Source: CAD feature listing. Evaluate the final solid. Frame: model axes, mm. A direction names the side the tool comes from. Give positions to 0.01 mm unless a question says otherwise; leave off trailing zeros. Loops run counter-clockwise (first coordinate to the right, second up) from the corner with the lowest first, then second, coordinate; pieces in that order, holes last. Notation, with made-up numbers: (-33, 66.25) - (-23, 66.25) arc R13 cw to (-23, 78.25) - close; hole circle Ø5 at (-10.5, 3.5). An arc over 180 degrees is marked (long way). Put each result on its own line as item: value.
Autodesk Inventor part; units mm, degrees
ref_plane "YZ Plane" through (0, 0, 0) normal (1, 0, 0) x (0, 1, 0)
ref_plane "XZ Plane" through (0, 0, 0) normal (0, 1, 0) x (-1, 0, 0)
ref_plane "XY Plane" through (0, 0, 0) normal (0, 0, 1) x (1, 0, 0)
sketch "Boceto1" plane through (0, 0, 0) normal (0, 1, 0) x (-1, 0, 0)
  circle A0 centre (0, 0) radius 30
  circle A1 centre (0, 0) radius 35
  dimension "d0" = 60
  dimension "d1" = 70
extrude "Extrusión1" add sketch "Boceto1" along normal blind 100
sketch "Boceto2" plane through (0, 0, 0) normal (0, -1, 0) x (1, 0, 0)
  line L0 (0, 0) -> (0, 45)
  line L1 (45, 35) -> (45, -35)
  line L2 (40, 35) -> (40, -35)
  line L3 (45, 0) -> (45, -35)
  line L4 (45, -35) -> (40, -35)
  line L5 (45, 0) -> (45, 35)
  line L6 (45, 35) -> (40, 35)
extrude "Extrusión2" add sketch "Boceto2" against normal blind 35
sketch "Boceto3" plane through (45, 0, 35) normal (1, 0, 0) x (0, 0, -1)
  line L0 (35, 0) -> (35, 35)
  circle A0 centre (35, 35) radius 35
  line L1 (0, 0) -> (0, 35)
  line L2 (0, 35) -> (0, 0)
  line L3 (70, 0) -> (0, 0)
  line L4 (0, 0) -> (70, 0)
  line L5 (70, 0) -> (70, 35)
  line L6 (70, 0) -> (70, 35)
  point P0 (70, 35)
extrude "Extrusión3" cut sketch "Boceto3" against normal blind 100 contours L5 L3 A0 | A0 L3 L1
sketch "Boceto4" plane through (45, 35, 0) normal (1, 0, 0) x (0, 0, -1)
  line L0 (-35, 0) -> (35, 0)
  line L1 (-35, 0) -> (35, 0)
  point P0 (0, -35)
sketch "Boceto5" plane through (0, 35, 0) normal (0, 1, 0) x (1, 0, 0)
  line L0 (40, 35) -> (40, -35)
  line L1 (40, -35) -> (45, -35)
  line L2 (40, -35) -> (45, -35)
  line L3 (45, -35) -> (45, 35)
  line L4 (45, -35) -> (45, 35)
  line L5 (45, 35) -> (40, 35)
  line L6 (45, 35) -> (40, 35)
  line L7 (40, 35) -> (40, -35)
  point P0 (0, 0)
extrude "Extrusión4" cut sketch "Boceto5" against normal blind 35
sketch "Boceto6" plane through (0, 100, 0) normal (0, 1, 0) x (1, 0, 0)
  circle A0 centre (0, 0) radius 42.5
  circle A1 centre (0, 0) radius 32.5
  dimension "d19" = 85
  dimension "d20" = 65
extrude "Extrusión5" add sketch "Boceto6" along normal blind 35
fillet "Empalme1" radius 30 1 edges at (35, 100, 0)
fillet "Empalme2" radius 2 1 edges at (-32.5, 100, 0)
fillet "Empalme3" radius 30 2 edges at (0, 100, -42.5) (0, 100, 42.5)
sketch "Boceto7" plane through (0, 135, 0) normal (0, 1, 0) x (1, 0, 0)
  circle A0 centre (0, 0) radius 32.5
  circle A1 centre (0, 0) radius 37.5
  dimension "d26" = 75
extrude "Extrusión6" cut sketch "Boceto7" against normal blind 30
properties part number "Modelo1_tronco_Pepu"
1) Pin query (flat end, axial travel): P1, Ø3, axis at x = -18, z = 25.5, coming from the -Y side; P2, Ø4, axis at x = -5, y = 72, coming from the +Z side; P3, Ø10, axis at x = 22.5, y = 49, coming from the +Z side. Return the tip coordinate at first contact, or that it passes through.
Check result:
P1: y = 9.52
P2: z = 34.87
P3: z = 30.31
2) Section query A-A, the plane y = 13.5. Output: boundary loops of the cut face in (x, z), plus the area to 3 significant figures.
Check result:
outline: (-21.5, -27.62) - (-11.72, -27.62) arc R30 cw to (-11.72, 27.62) - (-21.5, 27.62) arc R35 ccw to start; (11.72, -27.62) - (21.5, -27.62) arc R35 ccw to (21.5, 27.62) - (11.72, 27.62) arc R30 cw to start
area: 663 mm²
3) Section query B-B, the plane y = 116. Output: boundary loops of the cut face in (x, z).
Check result:
outline: circle Ø85 at (0, 0); hole circle Ø75 at (0, 0)
4) Material intervals for line 1 along Z through (x, y) = (0, 65); line 2 along Z through (x, y) = (0, 126.5), sorted ascending. Write a range as [from, to].
Check result:
line 1: [-35, -30], [30, 35]
line 2: [-42.5, -37.5], [37.5, 42.5]
5) Section query C-C, the plane y = 45. Output: boundary loops of the cut face in (x, z), plus the area to 3 significant figures.
Check result:
outline: circle Ø70 at (0, 0); hole circle Ø60 at (0, 0)
area: 1,020 mm²
6) Mould query, pull axis Z, two halves, no side actions, for faces 3 (the flat face through (0, 135, 38)), 4 (the cylindrical face through (-4.88, 120.21, -37.18)), 5 (the cylindrical face through (-32.33, 48.42, 13.41)). Classes: pulls with the +Z half, pulls with the -Z half, needs draft (parallel to the pull), parting line crosses it, or undercut.
Check result:
face 3: needs draft
face 4: undercut
face 5: parting line crosses it
7) Access query for faces 1 (the flat face through (-22.5, 100, -20.2)), 2 (the cylindrical face through (-20.58, 8.35, 22.69)). Directions: +Z, -Z, +X, -X, +Y, -Y. A direction counts if a zero-diameter tool reaches every point of the face in a straight line with its end or side. Return the directions, or none.
Check result:
face 1: +Y
face 2: +X, -X, -Y
